Autodesk Inventor part; units mm, degrees
ref_plane "YZ Plane" through (0, 0, 0) normal (1, 0, 0) x (0, 1, 0)
ref_plane "XZ Plane" through (0, 0, 0) normal (0, 1, 0) x (-1, 0, 0)
ref_plane "XY Plane" through (0, 0, 0) normal (0, 0, 1) x (1, 0, 0)
sketch "Skizze1" plane through (0, 0, 0) normal (0, 1, 0) x (-1, 0, 0)
  line L0 (0, 0) -> (10, 0)
  line L1 (10, 0) -> (10, -80)
  line L2 (10, -80) -> (0, -80)
  line L3 (0, -80) -> (0, 0)
  dimension "d0" = 10
  dimension "d1" = 80
extrude "Extrusion1" add sketch "Skizze1" along normal blind 20
sketch "Skizze2" plane through (0, 20, 0) normal (0, 1, 0) x (1, 0, 0)
  line L0 (0, 0) -> (-5, 0)
  line L1 (-10, 0) -> (0, 0)
  line L2 (-5, 0) -> (-5, 2.25)
  line L3 (-5, 2.25) -> (-5, 17.75)
  dimension "d4" = 2.25
  dimension "d5" = 15.5
hole "Bohrung1" at (-5, 20, -2.25) at (-5, 20, -17.75) direction (0, -1, 0) diameter 2 depth 8 tip angle 118
sketch "Skizze3" plane through (0, 0, 0) normal (1, 0, 0) x (0, 0, -1)
  line L0 (80, 0) -> (0, 0)
  line L1 (80, 0) -> (80, 10)
  line L2 (80, 0) -> (80, 20)
  line L3 (80, 10) -> (30, 10)
  line L4 (30, 10) -> (40, 10)
  line L5 (40, 10) -> (70, 10)
  dimension "d13" = 50
  dimension "d14" = 10
  dimension "d15" = 30
hole "Bohrung2" at (0, 10, -40) at (0, 10, -70) direction (-1, 0, 0) diameter 5 end through all
properties part number "Sensor_Halterung_Teil1" material "Holz (Eiche)"
Check sheet for the modelled part. Datum: model origin and axes. Units: mm. A direction names the side the tool comes from. Give positions to 0.01 mm unless a question says otherwise; leave off trailing zeros. Write each loop counter-clockwise with the first axis right and the second up, starting at its lowest first coordinate (ties: lowest second). Pieces come first, ordered by that corner, then holes. Notation, with made-up numbers: (35, 11) -> (59, 11) arc R23 ccw to (59, 23) -> close; hole circle Ø2 at (78.5, 32.5). An arc over 180 degrees is marked (long way). Use CSV: the item, a comma, the result in double quotes. Start each with the question number.
Q1. Release check for a two-part mould opening along Z. For faces 1 (the cylindrical face through (-5.3, 15.944, -16.796)), 2 (the flat face through (-5, 10, 0)), 3 (the flat face through (-10, 5, -39)) record: +Z half, -Z half, draft (parallel to the pull), parting line (faces both ways), or undercut.
Q2. Tool access check on faces 4 (the flat face through (-5, 0, -39)), 5 (the cylindrical face through (-5.99, 15.94, -2.38)). Record the directions out of +Z, -Z, +X, -X, +Y, -Y that give a thin tool (end or side, any length) a straight path to the whole face; none if there is none.
Q3. Cross-section at A-A on y = 10. Enter the section's corners in (x, z).
Q4. Scan lines: line 1 along Z through (x, y) = (-5, 17.75); line 2 along Z through (x, y) = (-5.25, 10); line 3 along X through (y, z) = (14.5, -17.75). Record each from-to range of solid material in increasing order.
Q5. Cross-section at B-B on z = -40. Enter the section's corners in (x, y).
Q6. Cross-section at C-C on x = -8.75. Enter the section's corners in (y, z).
Working result:
1,face 1,"undercut"
1,face 2,"+Z half"
1,face 3,"draft"
2,face 4,"+Z, -Z, +X, -X, -Y"
2,face 5,"+Y"
3,outline,"(-10, -80) -> (0, -80) -> (0, -72.5) -> (-10, -72.5) -> close; (-10, -67.5) -> (0, -67.5) -> (0, -42.5) -> (-10, -42.5) -> close; (-10, -37.5) -> (0, -37.5) -> (0, 0) -> (-10, 0) -> close"
4,line 1,"z = -80 to -18.75, -16.75 to -3.25, -1.25 to 0"
4,line 2,"z = -80 to -72.5, -67.5 to -42.5, -37.5 to 0"
4,line 3,"x = -10 to -6, -4 to 0"
5,outline,"(-10, 0) -> (0, 0) -> (0, 7.5) -> (-10, 7.5) -> close; (-10, 12.5) -> (0, 12.5) -> (0, 20) -> (-10, 20) -> close"
6,outline,"(0, -80) -> (20, -80) -> (20, 0) -> (0, 0) -> close; hole circle Ø5 at (10, -70); hole circle Ø5 at (10, -40)"
